The listing builds one solid part. Answer for the finished solid, in the listing's coordinates (mm). Coordinates: 2 decimals unless noted, no trailing zeros. Order: outer loops, then holes, each group sorted by start corner. A loop starts at its lowest first (then second) coordinate and runs counter-clockwise, first axis right, second up. Notation, with made-up numbers: (53, 1) -> (81, 1) arc R19 ccw to (81, 23) -> close; hole circle Ø6 at (-20, 28). An arc over 180 degrees is marked (long way). Write each question's results on one line, items separated by ' | '. Start each with the question number.
(1) Straight lines are drawn through the part: L1, parallel to Y at x = 2, z = 0; L2, parallel to X at y = 10, z = 22; L3, parallel to Y at x = -5, z = 12. For each, find the intervals that lie inside material, in ascending order.
(2) Given pin 1 (6 mm diameter, centred on x = -8, z = 27, fed in from -Y); pin 2 (3 mm diameter, centred on x = 10.5, y = -4.5, fed in from -Z); pin 3 (1 mm diameter, centred on y = -10, z = 24.5, fed in from -X); pin 4 (10 mm diameter, centred on x = -11, y = 6.5, fed in from +Z), each flat-ended and moving along its own axis, determine where each tip first touches the part or whether it passes through.
(3) The part is cut by section B-B, the plane x = -12. Give the vertices of the cut face in (y, z), then the cut area to 3 significant figures.
(4) The part is cut by section D-D, the plane y = -14. Give the vertices of the cut face in (x, z), then the cut area to 3 significant figures.
(5) The part is cut by section C-C, the plane z = -1. Give the vertices of the cut face in (x, y) (1 decimal).
(6) The part is cut by section A-A, the plane y = 2.5. Give the vertices of the cut face in (x, z).
```python
from build123d import *


with BuildPart() as f2:
    # F0 (on Top) → F2 (revolve)
    with BuildSketch(Plane.XY):
        with BuildLine():
            ThreePointArc((40, -46.1880215352), (54.6410161514, 8.4529946162), (0, 23.0940107676))
            Line((0, 23.0940107676), (20, -11.5470053838))
            Line((20, -11.5470053838), (40, -46.1880215352))
        make_face()
    revolve(axis=Axis((30, -28.8675134595, 0), (0.5, -0.8660254038, 0)))


with BuildPart() as f3:
    # F0 (on Top) → F3 (revolve)
    with BuildSketch(Plane.XY):
        with BuildLine():
            ThreePointArc((-60, -11.5470053838), (-20, -51.5470053838), (20, -11.5470053838))
            Line((20, -11.5470053838), (-20, -11.5470053838))
            Line((-20, -11.5470053838), (-60, -11.5470053838))
        make_face()
    revolve(axis=Axis((-40, -11.5470053838, 0), (-1, 0, 0)))


with BuildPart() as f4:
    # F0 (on Top) → F4 (revolve)
    with BuildSketch(Plane.XY):
        with BuildLine():
            Line((-20, -11.5470053838), (0, 23.0940107676))
            Line((0, 23.0940107676), (20, 57.735026919))
            ThreePointArc((20, 57.735026919), (-34.6410161514, 43.0940107676), (-20, -11.5470053838))
        make_face()
    revolve(axis=Axis((10, 40.4145188433, 0), (0.5, 0.8660254038, 0)))


with BuildPart() as f5:
    # F1 (on Right) → F5 (revolve)
    with BuildSketch(Plane.YZ):
        with BuildLine():
            Line((-23.0940107676, 65.3197264742), (0, 32.6598632371))
            Line((0, 32.6598632371), (23.0940107676, 0))
            ThreePointArc((23.0940107676, 0), (32.6598632371, 55.7538740047), (-23.0940107676, 65.3197264742))
        make_face()
    revolve(axis=Axis((0, -11.5470053838, 48.9897948557), (0, 0.5773502692, -0.8164965809)))


with BuildPart() as f2_1:
    add(f2.part)

    # F6: intersect F3, F4, F5
    add(f3.part, mode=Mode.INTERSECT)
    add(f4.part, mode=Mode.INTERSECT)
    add(f5.part, mode=Mode.INTERSECT)


solid = f2_1.part
```
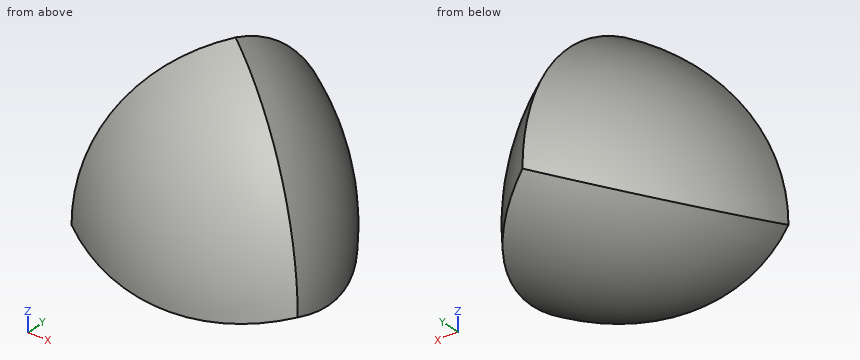
Established:
1) L1: y = -16.86 to 21.86 | L2: x = -5.53 to 5.53 | L3: y = -14.73 to 17.28
2) pin 1: stops at y = -8 | pin 2: stops at z = -6.09 | pin 3: passes through | pin 4: stops at z = 25.44
3) outline: (-14.99, -2.43) arc R38.16 ccw to (12.2, -3.5) arc R24 ccw to (-6.93, 23.55) arc R38.16 ccw to start | area: 600 mm^2
4) outline: (-14.87, -1.73) arc R37.47 ccw to (14.87, -1.73) arc R14.97 ccw (long way) to start | area: 465 mm^2
5) outline: (-19.9, -8.5) arc R21.6 ccw to (-17.3, -13) arc R40 ccw to (17.3, -13) arc R21.6 ccw to (19.9, -8.5) arc R40 ccw to (2.6, 21.5) arc R21.6 ccw to (-2.6, 21.5) arc R40 ccw to start
6) outline: (-17.31, -3.32) arc R39.92 ccw to (17.31, -3.32) arc R37.45 ccw to (0, 31.67) arc R37.45 ccw to start
